from build123d import *
from OCP.BRepFilletAPI import BRepFilletAPI_MakeChamfer

# Parameters (mm, degrees)
SKETCH_1_W          = 37
SKETCH_1_H          = 60
SKETCH_1_R          = 2.3
EXTRUDE_1_DEPTH     = 3
CHAMFER_1_SIZE      = 2
SKETCH_2_W          = 37
SKETCH_2_H          = 60
SKETCH_2_W_2        = 34
SKETCH_2_H_2        = 57
EXTRUDE_1_2_DEPTH   = 20
SKETCH_3_W          = 25
SKETCH_3_H          = 3.030341357
CUT_EXTRUDE_1_DEPTH = 20
SKETCH_4_R          = 2.5
EXTRUDE_2_DEPTH     = 20
SKETCH_5_R          = 1.55
CUT_EXTRUDE_2_DEPTH = 10
SKETCH_6_W          = 16
SKETCH_6_H          = 4
EXTRUDE_3_DEPTH     = 6
SKETCH_7_W          = 7.5
SKETCH_7_H          = 4.667229269
CUT_EXTRUDE_3_DEPTH = 1
FILLET_2_R          = 0.5
FILLET_3_R          = 2
CHAMFER_4_SIZE      = 0.866025404
CHAMFER_4_SIZE_2    = 1.5
FILLET_4_R          = 1
CHAMFER_5_SIZE      = 0.5
CHAMFER_5_SIZE_2    = 0.288675135
CHAMFER_6_SIZE      = 0.5
CHAMFER_6_SIZE2     = 0.288675135
FILLET_5_R          = 1


with BuildPart() as part:
    # Эскиз1 → Extrude 1 (new body)
    with BuildSketch(Plane(origin=(0, 0, 0), x_dir=(1, 0, 0), z_dir=(0, 1, 0))):
        Rectangle(SKETCH_1_W, SKETCH_1_H)
        with Locations(Location((0, 24, 0), (0, 0, 270))):
            Circle(SKETCH_1_R, mode=Mode.SUBTRACT)
        with Locations(Location((0, -24, 0), (0, 0, 270))):
            Circle(SKETCH_1_R, mode=Mode.SUBTRACT)
    extrude(amount=EXTRUDE_1_DEPTH)

    # Фаска1
    chamfer_1_edges = [part.edges().sort_by_distance(p)[0] for p in [
        (0, 3, -26.3),
        (0, 3, 21.7),
    ]]
    chamfer(chamfer_1_edges, length=CHAMFER_1_SIZE)

    # Эскиз2 → Extrude 1 2 (add)
    with BuildSketch(Plane(origin=(0, 3, 0), x_dir=(1, 0, 0), z_dir=(0, 1, 0))):
        Rectangle(SKETCH_2_W, SKETCH_2_H)
        Rectangle(SKETCH_2_W_2, SKETCH_2_H_2, mode=Mode.SUBTRACT)
    extrude(amount=EXTRUDE_1_2_DEPTH)

    # Эскиз3 → Вырез-Вытянуть1 (cut)
    with BuildSketch(Plane(origin=(0, 23, 0), x_dir=(1, 0, 0), z_dir=(0, 1, 0))):
        with Locations((0, 29.478101209)):
            Rectangle(SKETCH_3_W, SKETCH_3_H)
    extrude(amount=-CUT_EXTRUDE_1_DEPTH, mode=Mode.SUBTRACT)

    # Эскиз4 → Бобышка-Вытянуть2 (add)
    with BuildSketch(Plane(origin=(0, 3, 0), x_dir=(1, 0, 0), z_dir=(0, 1, 0))):
        with Locations((15, 18)):
            Circle(SKETCH_4_R)
        with Locations((-15, 18)):
            Circle(SKETCH_4_R)
        with Locations((15, -18)):
            Circle(SKETCH_4_R)
        with Locations((-15, -18)):
            Circle(SKETCH_4_R)
    extrude(amount=EXTRUDE_2_DEPTH)

    # Эскиз5 → Вырез-Вытянуть2 (cut)
    with BuildSketch(Plane(origin=(0, 23, 0), x_dir=(1, 0, 0), z_dir=(0, 1, 0))):
        with Locations(Location((15, 18, 0), (0, 0, 270))):
            Circle(SKETCH_5_R)
        with Locations(Location((15, -18, 0), (0, 0, 270))):
            Circle(SKETCH_5_R)
        with Locations(Location((-15, -18, 0), (0, 0, 270))):
            Circle(SKETCH_5_R)
        with Locations(Location((-15, 18, 0), (0, 0, 270))):
            Circle(SKETCH_5_R)
    extrude(amount=-CUT_EXTRUDE_2_DEPTH, mode=Mode.SUBTRACT)

    # Эскиз6 → Бобышка-Вытянуть3 (add)
    with BuildSketch(Plane(origin=(0, 3, 0), x_dir=(1, 0, 0), z_dir=(0, 1, 0))):
        with Locations((0, 4)):
            Rectangle(SKETCH_6_W, SKETCH_6_H)
    extrude(amount=EXTRUDE_3_DEPTH)

    # Эскиз7 → Вырез-Вытянуть3 (cut)
    with BuildSketch(Plane(origin=(0, 23, 0), x_dir=(1, 0, 0), z_dir=(0, 1, 0))):
        with Locations((0, -28.649225697)):
            Rectangle(SKETCH_7_W, SKETCH_7_H)
    extrude(amount=-CUT_EXTRUDE_3_DEPTH, mode=Mode.SUBTRACT)

    # Скругление2
    fillet_2_edges = [part.edges().sort_by_distance(p)[0] for p in [
        (-3.75, 22.5, 28.5),
        (3.75, 22.5, 28.5),
        (3.75, 22.5, 30),
        (-3.75, 22.5, 30),
    ]]
    fillet(fillet_2_edges, radius=FILLET_2_R)

    # Скругление3
    fillet_3_edges = [part.edges().sort_by_distance(p)[0] for p in [
        (18.5, 11.5, 30),
        (-18.5, 11.5, 30),
        (-18.5, 11.5, -30),
        (18.5, 11.5, -30),
    ]]
    fillet(fillet_3_edges, radius=FILLET_3_R)

    # Фаска4
    # the kernel refuses this chamfer: 1.5, 0.866025404 mm, written as the material it takes off along each edge
    with BuildSketch(Plane(origin=(0, 0, 24), x_dir=(0, 0, 1), z_dir=(-1, 0, 0))) as chamfer_4_piece_1:
        Polygon((2.3 + CHAMFER_4_SIZE, 0), (2.3, CHAMFER_4_SIZE_2), (2.3, 0), align=None)
    revolve(axis=Axis((0, 0, 24), (0, 1, 0)), mode=Mode.SUBTRACT)
    with BuildSketch(Plane(origin=(16.5, 0, -30), x_dir=(0, -0.01932676561270073, 0.999813220622208), z_dir=(-1, 0, 0))) as chamfer_4_piece_2:
        Polygon((CHAMFER_4_SIZE_2 * 0.999813220622, CHAMFER_4_SIZE_2 * 0.0193267656127), (-CHAMFER_4_SIZE * 0.0193267656079, CHAMFER_4_SIZE * 0.999813220373), (0, 0), align=None)
    extrude(amount=33, mode=Mode.SUBTRACT)
    with BuildSketch(Plane(origin=(-18.5, 0, -28), x_dir=(0.999813220622208, -0.01932676561270073, 0), z_dir=(0, 0, 1)), Plane(origin=(18.5, 0, 28), x_dir=(-0.999813220622208, -0.01932676561270073, 0), z_dir=(0, 0, -1))) as chamfer_4_piece_3:
        Polygon((CHAMFER_4_SIZE_2 * 0.999813220622, CHAMFER_4_SIZE_2 * 0.0193267656127), (-CHAMFER_4_SIZE * 0.0193267656079, CHAMFER_4_SIZE * 0.999813220373), (0, 0), align=None)
    extrude(amount=56, mode=Mode.SUBTRACT)
    with BuildSketch(Plane(origin=(-16.5, 0, 30), x_dir=(0, 0.9983227437537924, 0.0578938624026721), z_dir=(1, 0, 0))) as chamfer_4_piece_4:
        Polygon((CHAMFER_4_SIZE * 0.998322743505, -CHAMFER_4_SIZE * 0.0578938623883), (-CHAMFER_4_SIZE_2 * 0.0578938624027, -CHAMFER_4_SIZE_2 * 0.998322743754), (0, 0), align=None)
    extrude(amount=33, mode=Mode.SUBTRACT)
    with BuildSketch(Plane(origin=(-16.5, 0, -28), x_dir=(0, 0, -1), z_dir=(1, 0, 0))) as chamfer_4_piece_5:
        Polygon((2 - CHAMFER_4_SIZE_2, 0), (2, CHAMFER_4_SIZE), (2, 0), align=None)
    revolve(axis=Axis((-16.5, 0, -28), (0, 1, 0)), revolution_arc=90, mode=Mode.SUBTRACT)
    with BuildSketch(Plane(origin=(-16.5, 0, 28), x_dir=(0, 0, 1), z_dir=(1, 0, 0))) as chamfer_4_piece_6:
        Polygon((2 - CHAMFER_4_SIZE_2, 0), (2, -CHAMFER_4_SIZE), (2, 0), align=None)
    revolve(axis=Axis((-16.5, 0, 28), (0, -1, 0)), revolution_arc=90, mode=Mode.SUBTRACT)
    with BuildSketch(Plane(origin=(16.5, 0, 28), x_dir=(0, 0, 1), z_dir=(-1, 0, 0))) as chamfer_4_piece_7:
        Polygon((2, CHAMFER_4_SIZE), (2 - CHAMFER_4_SIZE_2, 0), (2, 0), align=None)
    revolve(axis=Axis((16.5, 0, 28), (0, 1, 0)), revolution_arc=90, mode=Mode.SUBTRACT)
    with BuildSketch(Plane(origin=(16.5, 0, -28), x_dir=(0, 0, -1), z_dir=(-1, 0, 0))) as chamfer_4_piece_8:
        Polygon((2 - CHAMFER_4_SIZE_2, 0), (2, -CHAMFER_4_SIZE), (2, 0), align=None)
    revolve(axis=Axis((16.5, 0, -28), (0, -1, 0)), revolution_arc=90, mode=Mode.SUBTRACT)
    with BuildSketch(Plane(origin=(0, 0, -24), x_dir=(0, 0, 1), z_dir=(-1, 0, 0))) as chamfer_4_piece_9:
        Polygon((2.3 + CHAMFER_4_SIZE, 0), (2.3, CHAMFER_4_SIZE_2), (2.3, 0), align=None)
    revolve(axis=Axis((0, 0, -24), (0, 1, 0)), mode=Mode.SUBTRACT)

    # Скругление4
    fillet_4_edges = [part.edges().sort_by_distance(p)[0] for p in [
        (-8, 3, -4),
        (-8, 6, -6),
        (0, 3, -2),
        (-8, 6, -2),
        (8, 3, -4),
        (8, 6, -2),
        (0, 3, -6),
        (8, 6, -6),
        (-8, 9, -4),
        (8, 9, -4),
    ]]
    fillet(fillet_4_edges, radius=FILLET_4_R)

    # Фаска5
    # the kernel refuses this chamfer: 0.5, 0.288675135 mm, written as the material it takes off along each edge
    with BuildSketch(Plane(origin=(-8.293542877, 9, -6), x_dir=(0, -0.9998132206222079, -0.019326765612700324), z_dir=(1, 0, 0)), Plane(origin=(8.293542877, 9, -2), x_dir=(0, -0.9998132206222079, 0.01932676561270075), z_dir=(-1, 0, 0))) as chamfer_5_piece_1:
        Polygon((CHAMFER_5_SIZE * 0.999813220622, -CHAMFER_5_SIZE * 0.0193267656127), (-CHAMFER_5_SIZE_2 * 0.0193267655856, -CHAMFER_5_SIZE_2 * 0.999813219219), (0, 0), align=None)
    extrude(amount=16.587085755, mode=Mode.SUBTRACT)

    # Фаска6: one chamfer whose edges measure the first distance from different faces: ONE call of the kernel's chamfer builder (chamfer() names one face for all edges)
    chamfer_6_edges_1 = [part.edges().sort_by_distance(p)[0] for p in [
        (-15, 23, -19.55),
        (-15, 23, 16.45),
    ]]
    chamfer_6_side_1 = [part.faces().sort_by_distance(p)[0] for p in [
        (-10.375, 23, 29.382135735),
    ]]
    chamfer_6_edges_2 = [part.edges().sort_by_distance(p)[0] for p in [
        (15, 23, 16.45),
        (15, 23, -19.55),
    ]]
    chamfer_6_side_2 = [part.faces().sort_by_distance(p)[0] for p in [
        (10.375, 23, 29.382135735),
    ]]
    chamfer_6 = BRepFilletAPI_MakeChamfer(part.part.solid().wrapped)
    for e in chamfer_6_edges_1:
        chamfer_6.Add(CHAMFER_6_SIZE, CHAMFER_6_SIZE2, e.wrapped, chamfer_6_side_1[0].wrapped)  # the first distance lies on this face
    for e in chamfer_6_edges_2:
        chamfer_6.Add(CHAMFER_6_SIZE, CHAMFER_6_SIZE2, e.wrapped, chamfer_6_side_2[0].wrapped)  # the first distance lies on this face
    add(Compound.cast(chamfer_6.Shape()), mode=Mode.REPLACE)

    # Скругление5
    fillet_5_edges = [part.edges().sort_by_distance(p)[0] for p in [
        (0, 3, -30),
        (-12.5, 13, -30),
        (12.5, 13, -30),
    ]]
    fillet(fillet_5_edges, radius=FILLET_5_R)


solid = part.part
The model under review builds one solid part; all positions refer to its coordinate system, in mm. A direction names the side the tool comes from. Give positions to 0.01 mm unless a question says otherwise; leave off trailing zeros. Loops run counter-clockwise (first coordinate to the right, second up) from the corner with the lowest first, then second, coordinate; pieces in that order, holes last. Notation, with made-up numbers: (10.25, -23) -> (55.25, -23) arc R4 ccw to (55.25, -18) -> close; hole circle Ø9 at (12.5, 46). An arc over 180 degrees is marked (long way). Write each question's results on one line, items separated by ' | '.
1) Draft analysis for pull direction Z (two halves, no side actions). For faces 1 (the face through (-17.26, 0.34, 28.78)), 2 (the face through (-13.69, 17.92, -17.17)), 3 (the face through (0, 6, -6)), state which applies: pulls with the +Z half, pulls with the -Z half, needs draft (parallel to the pull), parting line crosses it, or undercut.
Conclusion:
face 1: pulls with the +Z half | face 2: undercut | face 3: pulls with the -Z half
2) For line 1 along Z through (x, y) = (-15, 8.75); line 2 along X through (y, z) = (15, -18); line 3 along X through (y, z) = (18.5, 24.5), list the stretches that pass through material, from the lowest coordinate up. Write a range as from..to.
Conclusion:
line 1: z = -30..-28.5, -20.5..-15.5, 15.5..20.5, 28.5..30 | line 2: x = -18.5..-16.55, -13.45..-12.5, 12.5..13.45, 16.55..18.5 | line 3: x = -18.5..-17, 17..18.5
3) Take a section at B-B, the plane z = -18. Give the boundary of the cut face in (x, y), plus the area to 3 significant figures.
Conclusion:
outline: (-18.5, 0.87) -> (-17, 0) -> (17, 0) -> (18.5, 0.87) -> (18.5, 23) -> (17.05, 23) -> (16.55, 22.71) -> (16.55, 13) -> (13.45, 13) -> (13.45, 22.71) -> (12.95, 23) -> (12.5, 23) -> (12.5, 3) -> (-12.5, 3) -> (-12.5, 23) -> (-12.95, 23) -> (-13.45, 22.71) -> (-13.45, 13) -> (-16.55, 13) -> (-16.55, 22.71) -> (-17.05, 23) -> (-18.5, 23) -> close | area: 287 mm^2
4) Take a section at D-D, the plane z = 24. Give the boundary of the cut face in (x, y), plus the area to 3 significant figures.
Conclusion:
outline: (-18.5, 0.87) -> (-17, 0) -> (-3.17, 0) -> (-2.48, 1.18) -> (-4.3, 3) -> (-17, 3) -> (-17, 23) -> (-18.5, 23) -> close; (2.48, 1.18) -> (3.17, 0) -> (17, 0) -> (18.5, 0.87) -> (18.5, 23) -> (17, 23) -> (17, 3) -> (4.3, 3) -> close | area: 151 mm^2
5) Insertion check: pin 1 Ø1.2 at (x, z) = (0, 29) entering from +Y; pin 2 Ø3.5 at (x, z) = (-15.5, -18.5) entering from +Y; pin 3 Ø2 at (x, z) = (-0.5, -9) entering from +Y; pin 4 Ø0.6 at (y, z) = (22.5, 29) entering from -X. Each pin has a flat end and moves straight along its axis. Give the tip position at first contact, or say it passes through.
Conclusion:
pin 1: stops at y = 22 | pin 2: stops at y = 23 | pin 3: stops at y = 3 | pin 4: stops at x = -18.37
6) Take a section at A-A, the plane y = 14. Count the separate pieces of the cut face and the enclosed holes in it, plus the area to 3 significant figures.
Conclusion:
separate pieces: 1 | enclosed holes: 4 | area: 285 mm^2
7) Tool access review of faces 4 (the face through (15, 13, -18)), 5 (the face through (8, 6, -4)), 6 (the face through (18.5, 12, 0)): name each direction out of +Z, -Z, +X, -X, +Y, -Y from which nothing blocks a thin tool from reaching the whole face with its end or side.
Conclusion:
face 4: +Y | face 5: -Z, +Y | face 6: +Z, -Z, +X, +Y, -Y
